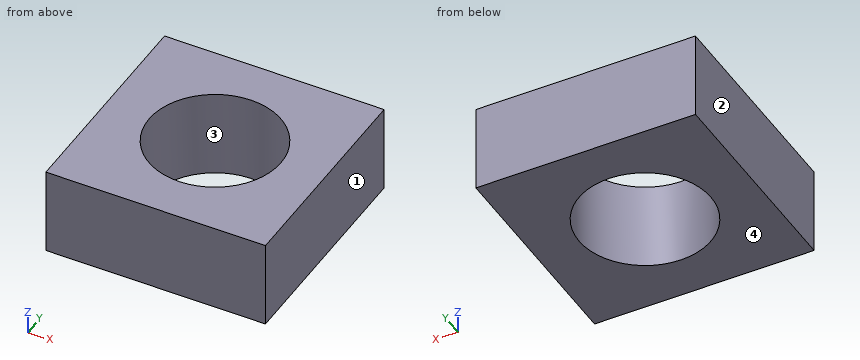
```python
from build123d import *

# Parameters (mm, degrees)
F0_W     = 25
F0_H     = 25
F1_DEPTH = 10
F2_R     = 7.5
F3_DEPTH = 10.001


with BuildPart() as f1:
    # F0 (on Top) → F1 (new body)
    with BuildSketch(Plane.XY):
        with Locations((3.349018, -9.797464)):
            Rectangle(F0_W, F0_H)
    extrude(amount=F1_DEPTH)

    # F2 (on face) → F3 (cut, through all)
    with BuildSketch(Plane(origin=(0, 0, 0), x_dir=(1, 0, 0), z_dir=(0, 0, -1))):
        with Locations((3.349018, 9.797464)):
            Circle(F2_R)
    extrude(amount=-F3_DEPTH, mode=Mode.SUBTRACT)


solid = f1.part
```
Verification items for the finished model (mm, model axes). Face numbers are marked on the shaded views. Coordinates: 2 decimals unless noted, no trailing zeros. Write each loop counter-clockwise with the first axis right and the second up, starting at its lowest first coordinate (ties: lowest second). Pieces come first, ordered by that corner, then holes. Notation, with made-up numbers: M -15.5,1 L 32.5,1 A34 ccw 32.5,35 Z; hole C 86,62 d2. An arc over 180 degrees is marked long. Answer as a JSON object with one key per item and string values. Group by question number.
(1) Cross-section at A-A, the plane x = 5.75. Record the cut outline in (y, z), and give its area (3 significant figures).
(2) Material ranges on line 1 (X direction, y = -10, z = 4.5); line 2 (Y direction, x = 3, z = 5); line 3 (X direction, y = -16, z = 5.25), recorded low to high.
(3) Cross-section at C-C, the plane z = 8. Record the cut outline in (x, y).
(4) Cross-section at B-B, the plane y = -17. Record the cut outline in (x, z).
(5) Release check for a two-part mould opening along X. For the marked faces 1, 2, 3 and 4 record: +X half, -X half, draft (parallel to the pull), parting line (faces both ways), or undercut.
(6) Gauge pin test, flat end, axial feed: pin 1 (6 mm diameter, centred on x = 2, y = -9, fed in from -Z). Record the tip position at first contact, or that the pin passes through.
Reply:
{
 "1": {"outline": "M -22.3,0 L -16.9,0 L -16.9,10 L -22.3,10 Z; M -2.69,0 L 2.7,0 L 2.7,10 L -2.69,10 Z", "area": "108 mm²"},
 "2": {"line 1": "-9.15 to -4.15, 10.85 to 15.85", "line 2": "-22.3 to -17.29, -2.31 to 2.7", "line 3": "-9.15 to -0.87, 7.57 to 15.85"},
 "3": {"outline": "M -9.15,-22.3 L 15.85,-22.3 L 15.85,2.7 L -9.15,2.7 Z; hole C 3.35,-9.8 d15"},
 "4": {"outline": "M -9.15,0 L 1.26,0 L 1.26,10 L -9.15,10 Z; M 5.44,0 L 15.85,0 L 15.85,10 L 5.44,10 Z"},
 "5": {"face 1": "+X half", "face 2": "-X half", "face 3": "undercut", "face 4": "draft"},
 "6": {"pin 1": "through"}
}
